```python
from build123d import *

# Parameters (mm, degrees)
F0_R          = 5
F1_DEPTH      = 100
F2_R          = 2.5
F3_DEPTH      = 2.5
F3_DEPTH_BACK = 102.5


with BuildPart() as f1:
    # F0 (on Front) → F1 (new body)
    with BuildSketch(Plane.XZ):
        Circle(F0_R)
    extrude(amount=F1_DEPTH)

    # F2 (on face) → F3 (join, two sides)
    with BuildSketch(Plane.XZ.offset(100)) as f3_sk:
        Circle(F2_R)
    extrude(amount=F3_DEPTH)
    extrude(f3_sk.sketch, amount=-F3_DEPTH_BACK)


solid = f1.part
```
Input: part model. Units: mm. Frame: model coordinates. A direction names the side the tool comes from. Round coordinates to 2 decimals unless told otherwise and drop trailing zeros. Loops run counter-clockwise (first coordinate to the right, second up) from the corner with the lowest first, then second, coordinate; pieces in that order, holes last. Notation, with made-up numbers: M -7,27.25 L 15,27.25 A12 ccw 15,46.25 Z; hole C 49.25,-36 d7. An arc over 180 degrees is marked long. Answer in a Markdown table with one row per item. Add a question column.
1. Ray query, probe 1 along Y at (x, z) = (-3.25, 3); probe 2 along X at (y, z) = (-16, 1.75); probe 3 along Z at (x, y) = (-2.5, -21). Return the intervals inside material, ascending.
2. Section D-D (x = 3.75). Output: boundary loops of the cut face in (y, z), and give its area (3 significant figures).
3. Section A-A (x = 0). Output: boundary loops of the cut face in (y, z), and give its area (4 significant figures).
4. Section C-C (y = -10). Output: boundary loops of the cut face in (x, z).
5. Contact query for flat-ended pins moving along their axis: pin 1 (6 mm diameter, centred on x = 3.5, y = -8, fed in from -Z); pin 2 (1.5 mm diameter, centred on x = 0.5, z = -3.5, fed in from +Y); pin 3 (2 mm diameter, centred on y = -56, z = -3.5, fed in from +X). Output: stop coordinate, or through.
6. Set-up query: faces 1 (the face through (-0.54, -101.23, -2.44)), 2 (the face through (-0.54, 1.23, -2.44)), 3 (the face through (0, 2.5, 0)). Return all of +Z, -Z, +X, -X, +Y, -Y with unobstructed straight access to the full face (end or side cutting, diameter ignored); none if empty.
7. Section B-B (z = 0). Output: boundary loops of the cut face in (x, y).
Values follow:
| question | item | result |
|---|---|---|
| 1 | probe 1 | -100 to 0 |
| 1 | probe 2 | -4.68 to 4.68 |
| 1 | probe 3 | -4.33 to 4.33 |
| 2 | outline | M -100,-3.31 L 0,-3.31 L 0,3.31 L -100,3.31 Z |
| 2 | area | 661 mm^2 |
| 3 | outline | M -102.5,-2.5 L -100,-2.5 L -100,-5 L 0,-5 L 0,-2.5 L 2.5,-2.5 L 2.5,2.5 L 0,2.5 L 0,5 L -100,5 L -100,2.5 L -102.5,2.5 Z |
| 3 | area | 1,025 mm^2 |
| 4 | outline | C 0,0 d10 |
| 5 | pin 1 | z = -4.97 |
| 5 | pin 2 | y = 0 |
| 5 | pin 3 | x = 4.33 |
| 6 | face 1 | -Y |
| 6 | face 2 | +Y |
| 6 | face 3 | +Z, -Z, +X, -X, +Y |
| 7 | outline | M -5,-100 L -2.5,-100 L -2.5,-102.5 L 2.5,-102.5 L 2.5,-100 L 5,-100 L 5,0 L 2.5,0 L 2.5,2.5 L -2.5,2.5 L -2.5,0 L -5,0 Z |
